Here's the drawing with two shaded views (mm, measured from the low corner). I have some questions. A direction names the side the tool comes from. Give positions to 0.01 mm unless a question says otherwise; leave off trailing zeros. Order: outer loops, then holes, each group sorted by start corner. A loop starts at its lowest first (then second) coordinate and runs counter-clockwise, first axis right, second up. Notation, with made-up numbers: (72, 75) - (131, 75) arc R27 ccw to (131, 109) - close; hole circle Ø2 at (-1.5, 38.5). An arc over 180 degrees is marked (long way). Use one line per item in the form item = value. Start each with the question number.
1) Please list where these lines run through material, in increasing order: probe 1 along Y at (x, z) = (35, 0.75); probe 2 along X at (y, z) = (37.7, 0.7).
2) We'd pull the mould along Y, two halves only. Please class the marked faces 4, 5 and 6: released by +Y, released by -Y, zero draft, split by the parting line, or undercut.
3) Suppose I cut it at A-A, the plane x = 52.5. Write out the boundary of the cut face in (y, z).
4) Suppose I cut it at B-B, the plane y = 18. Write out the boundary of the cut face in (x, z), and give its area (3 significant figures).
5) Suppose I cut it at C-C, the plane z = 4. State how many separate pieces and enclosed holes the cut face has, and give its area (3 significant figures).
6) For pin 1 (1 mm diameter, centred on y = 41, z = 5, fed in from -X); pin 2 (5.5 mm diameter, centred on x = 35, y = 12.3, fed in from +Z), each with a flat end and sliding along its axis, tell me the tip position at first contact or that it passes through.
7) Which directions (+Z, -Z, +X, -X, +Y, -Y) give clear straight access to the entire face, cutting with the end or side of a thin tool? Please do the marked faces 1, 2 and 3.
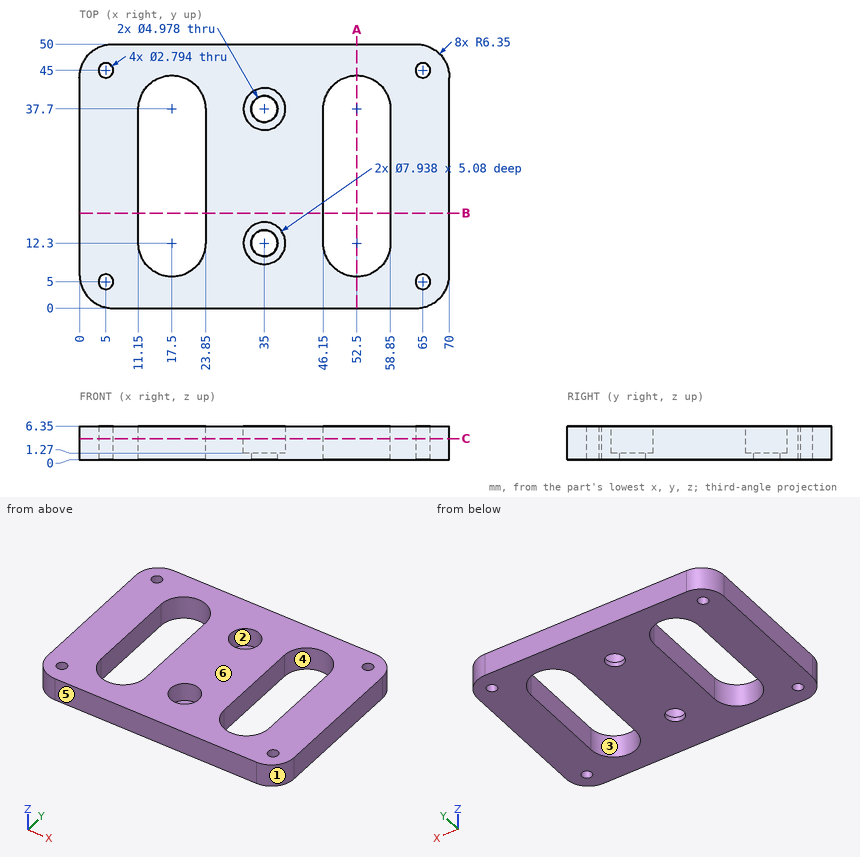
Result sheet:
q1.probe_1 = 0 to 9.81, 14.79 to 35.21, 40.19 to 50
q1.probe_2 = 0 to 11.15, 23.85 to 32.51, 37.49 to 46.15, 58.85 to 70
q2.face_4 = undercut
q2.face_5 = released by -Y
q2.face_6 = zero draft
q3.outline = (0, 0) - (5.95, 0) - (5.95, 6.35) - (0, 6.35) - close; (44.05, 0) - (50, 0) - (50, 6.35) - (44.05, 6.35) - close
q4.outline = (0, 0) - (11.15, 0) - (11.15, 6.35) - (0, 6.35) - close; (23.85, 0) - (46.15, 0) - (46.15, 6.35) - (23.85, 6.35) - close; (58.85, 0) - (70, 0) - (70, 6.35) - (58.85, 6.35) - close
q4.area = 283 mm²
q5.separate_pieces = 1
q5.enclosed_holes = 8
q5.area = 2,440 mm²
q6.pin_1 = 0
q6.pin_2 = 1.27
q7.face_1 = +Z, -Z, +X, -Y
q7.face_2 = +Z
q7.face_3 = +Z, -Z
